Autodesk Inventor part; units mm, degrees
ref_plane "YZ Plane" through (0, 0, 0) normal (1, 0, 0) x (0, 1, 0)
ref_plane "XZ Plane" through (0, 0, 0) normal (0, 1, 0) x (-1, 0, 0)
ref_plane "XY Plane" through (0, 0, 0) normal (0, 0, 1) x (1, 0, 0)
sketch "Sketch1" plane through (0, 0, 0) normal (0, 1, 0) x (-1, 0, 0)
  point P0 (0, 0)
sketch "Sketch2" plane through (0, 0, 0) normal (0, 1, 0) x (-1, 0, 0)
  line L0 (0, 0) -> (0, -70)
  line L1 (0, -70) -> (54.3409, -70) construction
  line L2 (0, -70) -> (60.6218, -105)
  line L3 (0, -70) -> (70, -70) construction
  line L4 (60.6218, -105) -> (121.2436, -70)
  line L5 (121.2436, -70) -> (121.2436, 0)
  line L6 (121.2436, 0) -> (60.6218, 35)
  line L7 (60.6218, 35) -> (0, 0)
  dimension "d0" = 70
  dimension "d2" = 70
  dimension "d3" = 30
  dimension "d4" = 70
  dimension "d5" = 120
  dimension "d6" = 70
  dimension "d7" = 120
extrude "Extrusion1" add sketch "Sketch2" along normal blind 3
sketch "Sketch3" plane through (0, 3, 0) normal (0, 1, 0) x (1, 0, 0)
  line L0 (0, 0) -> (0, 70)
  line L1 (-121.2436, 0) -> (-60.6218, -35)
  line L2 (-90.9327, -17.5) -> (-50.9327, -17.5) construction
  line L3 (-60.6218, 105) -> (-121.2436, 70)
  line L4 (-90.9327, 87.5) -> (-50.9327, 87.5) construction
  line L5 (-70.9327, 17.141) -> (-90.9327, -17.5) construction
  line L6 (-73.5307, 18.641) -> (-93.5307, -16)
  line L7 (-88.3346, -19) -> (-68.3346, 15.641)
  arc A0 (-68.3346, 15.641) -> (-73.5307, 18.641) centre (-70.9327, 17.141) ccw
  arc A1 (-93.5307, -16) -> (-88.3346, -19) centre (-90.9327, -17.5) ccw
  line L8 (-70.9327, 52.859) -> (-90.9327, 87.5) construction
  line L9 (-68.3346, 54.359) -> (-88.3346, 89)
  line L10 (-93.5307, 86) -> (-73.5307, 51.359)
  arc A2 (-73.5307, 51.359) -> (-68.3346, 54.359) centre (-70.9327, 52.859) ccw
  arc A3 (-88.3346, 89) -> (-93.5307, 86) centre (-90.9327, 87.5) ccw
  line L11 (-40, 35) -> (0, 35) construction
  line L12 (-40, 32) -> (0, 32)
  line L13 (0, 38) -> (-40, 38)
  arc A4 (-40, 38) -> (-40, 32) centre (-40, 35) ccw
  arc A5 (0, 32) -> (0, 38) centre (0, 35) ccw
  point P0 (-80.9327, -0.1795)
  point P1 (-80.9327, 70.1795)
  point P2 (-20, 35)
  dimension "d10" = 40
  dimension "d11" = 40
  dimension "d13" = 40
  dimension "d15" = 6
  dimension "d16" = 6
  dimension "d17" = 6
extrude "Extrusion3" cut sketch "Sketch3" against normal blind 3
sketch "Sketch4" plane through (0, 3, 0) normal (0, 1, 0) x (1, 0, 0)
  line L0 (-54, 7) -> (-54, 13) construction
  line L1 (-53.25, 7) -> (-53.25, 13)
  line L2 (-54.75, 13) -> (-54.75, 7)
  arc A0 (-54.75, 7) -> (-53.25, 7) centre (-54, 7) ccw
  arc A1 (-53.25, 13) -> (-54.75, 13) centre (-54, 13) ccw
  line L3 (-54, 10) -> (-48, 10) construction
  line L4 (-12, 7) -> (-12, 13) construction
  line L5 (-11.25, 7) -> (-11.25, 13)
  line L6 (-12.75, 13) -> (-12.75, 7)
  arc A2 (-12.75, 7) -> (-11.25, 7) centre (-12, 7) ccw
  arc A3 (-11.25, 13) -> (-12.75, 13) centre (-12, 13) ccw
  line L7 (-12, 10) -> (-6, 10) construction
  arc A4 (-40, 38) -> (-40, 32) centre (-40, 35) ccw
  line L8 (-121.2436, 70) -> (-121.2436, 0)
  arc A5 (-73.5307, 51.359) -> (-68.3346, 54.359) centre (-70.9327, 52.859) ccw
  line L9 (-60.6218, -35) -> (0, 0)
  line L10 (-42.282, 53.2346) -> (-45.282, 58.4308) construction
  line L11 (-39.684, 54.7346) -> (-44.8801, 51.7346) construction
  arc A6 (-45.2551, 52.3841) -> (-44.5051, 51.0851) centre (-44.8801, 51.7346) ccw
  line L12 (-44.5051, 51.0851) -> (-39.309, 54.0851)
  arc A7 (-39.309, 54.0851) -> (-40.059, 55.3841) centre (-39.684, 54.7346) ccw
  line L13 (-40.059, 55.3841) -> (-45.2551, 52.3841)
  line L14 (-65.5051, 87.4582) -> (-60.309, 90.4582)
  arc A8 (-60.309, 90.4582) -> (-61.059, 91.7572) centre (-60.684, 91.1077) ccw
  arc A9 (-66.2551, 88.7572) -> (-65.5051, 87.4582) centre (-65.8801, 88.1077) ccw
  line L15 (-60.684, 91.1077) -> (-65.8801, 88.1077) construction
  line L16 (-61.059, 91.7572) -> (-66.2551, 88.7572)
  line L17 (-63.282, 89.6077) -> (-66.282, 94.8038) construction
  line L18 (-85.5833, 41.7654) -> (-88.5833, 36.5692) construction
  line L19 (-88.1814, 43.2654) -> (-82.9852, 40.2654) construction
  arc A10 (-83.3602, 39.6159) -> (-82.6102, 40.9149) centre (-82.9852, 40.2654) ccw
  line L20 (-82.6102, 40.9149) -> (-87.8064, 43.9149)
  arc A11 (-87.8064, 43.9149) -> (-88.5564, 42.6159) centre (-88.1814, 43.2654) ccw
  line L21 (-88.5564, 42.6159) -> (-83.3602, 39.6159)
  line L22 (-103.6102, 4.5418) -> (-108.8064, 7.5418)
  arc A12 (-108.8064, 7.5418) -> (-109.5564, 6.2428) centre (-109.1814, 6.8923) ccw
  arc A13 (-104.3602, 3.2428) -> (-103.6102, 4.5418) centre (-103.9852, 3.8923) ccw
  line L23 (-109.1814, 6.8923) -> (-103.9852, 3.8923) construction
  line L24 (-109.5564, 6.2428) -> (-104.3602, 3.2428)
  line L25 (-106.5833, 5.3923) -> (-109.5833, 0.1962) construction
  point P0 (-60.6218, 35)
  dimension "d25" = 3
  dimension "d27" = 1.5
  dimension "d29" = 3
  dimension "d31" = 1.5
  dimension "d48" = 360
extrude "Extrusion4" cut sketch "Sketch4" against normal blind 10
sketch "Sketch5" plane through (0, 0, 0) normal (0, -1, 0) x (1, 0, 0)
  arc A0 (-73.5307, -18.641) -> (-68.3346, -15.641) centre (-70.9327, -17.141) ccw
  line L0 (-70.9327, -17.141) -> (-50.3109, -17.141) construction
  arc A1 (-40, -32) -> (-40, -38) centre (-40, -35) ccw
  point P0 (0, 0)
  point P1 (-60.6218, -35)
sketch "Sketch6" plane through (0, 3, 0) normal (0, 1, 0) x (1, 0, 0)
  line L0 (-60.6218, -35) -> (0, 0)
  circle A0 centre (-60.6218, -15) radius 1.4
  circle A1 centre (-17.3205, 60) radius 1.4
  circle A2 centre (-103.923, 60) radius 1.4
  circle A3 centre (-60.6218, 35) radius 1.4
  dimension "d52" = 2.8
  dimension "d55" = 360
  dimension "d57" = 2.8
extrude "Extrusion5" cut sketch "Sketch6" against normal blind 10
properties part number "servo mount"
Read the model definition and answer for the solid it produces. Units are mm, in the model's axes. A direction names the side the tool comes from. Coordinates: 2 decimals unless noted, no trailing zeros. Loops run counter-clockwise (first coordinate to the right, second up) from the corner with the lowest first, then second, coordinate; pieces in that order, holes last. Notation, with made-up numbers: (87, 75) -> (132, 75) arc R17 cw to (132, 83) -> close; hole circle Ø1 at (79.5, -1.5). An arc over 180 degrees is marked (long way). Return JSON: item names as keys, results as strings.
Item 1: Flat-ended cylindrical pins translate along their axes: P1, Ø1.7, axis at x = -103.923, z = -60, coming from the -Y side; P2, Ø1.5, axis at x = -14.5, y = 2, coming from the +Z side. Find the tip coordinate at first contact, or state that the pin passes through.
Answers:
{"P1": "passes through", "P2": "stops at z = 8.8"}
Item 2: Find the intervals of material crossed by probe 1 along Z at (x, y) = (-12, 1.4); probe 2 along X at (y, z) = (1.4, -60); probe 3 along X at (y, z) = (1.15, -35), in increasing order.
Answers:
{"probe 1": "z = -76.93 to -38, -32 to -13.75, -6.25 to 6.93", "probe 2": "x = -121.24 to -105.32, -102.52 to -78.52, -71.59 to -18.72, -15.92 to 0", "probe 3": "x = -121.24 to -62.02, -59.22 to -43"}
Item 3: Find section D-D (z = -94.5). Determine the outline of the cut face in (x, y).
Answers:
{"outline": "(-78.81, 0) -> (-42.44, 0) -> (-42.44, 3) -> (-78.81, 3) -> close"}
Item 4: For faces 4 (the flat face through (-29.887, 1.479, -87.255)), 5 (the flat face through (-78.475, 1.521, 1.922)), 6 (the flat face through (-20, 2, -32)), determine the directions among +Z, -Z, +X, -X, +Y, -Y from which every point of the face is accessible in a straight line to the end or side of a thin tool.
Answers:
{"face 4": "-Z, +X, +Y, -Y", "face 5": "+Y, -Y", "face 6": "+X, +Y, -Y"}
Item 5: For a pull along Z with two mould halves and no side action, classify faces 1 (the flat face through (0, 1, -16)), 2 (the flat face through (-106.99, 1.52, -4.76)), 3 (the flat face through (-107.193, 1.479, -78.112)) as +Z half, -Z half, draft (parallel to the pull), parting line (faces both ways), or undercut.
Answers:
{"face 1": "draft", "face 2": "undercut", "face 3": "-Z half"}
Item 6: Find section A-A (x = -22). Determine the outline of the cut face in (y, z).
Answers:
{"outline": "(0, -82.7) -> (3, -82.7) -> (3, -38) -> (0, -38) -> close; (0, -32) -> (3, -32) -> (3, 12.7) -> (0, 12.7) -> close"}
Item 7: Find section B-B (z = 2). Determine the outline of the cut face in (x, y), plus the area to 3 significant figures.
Answers:
{"outline": "(-117.78, 0) -> (-85.45, 0) -> (-85.45, 3) -> (-117.78, 3) -> close; (-78.52, 0) -> (-3.46, 0) -> (-3.46, 3) -> (-78.52, 3) -> close", "area": "322 mm2"}
Item 8: Find section C-C (y = 1.1). Count the separate pieces of the cut face and the enclosed holes in it, plus the area to 3 significant figures.
Answers:
{"separate pieces": "1", "enclosed holes": "10", "area": "11,900 mm2"}
